```python
from build123d import *

# Parameters (mm, degrees)
SKETCH1_R           = 25.4
SKETCH1_R_2         = 1.5
SKETCH1_R_3         = 12.7
BOSS_EXTRUDE1_DEPTH = 0.396875


with BuildPart() as part:
    # Sketch1 → Boss-Extrude1 (new body)
    with BuildSketch(Plane.XY):
        Circle(SKETCH1_R)
        with Locations((-15.5, 0)):
            Circle(SKETCH1_R_2, mode=Mode.SUBTRACT)
        with Locations((-7.75, 13.423393759)):
            Circle(SKETCH1_R_2, mode=Mode.SUBTRACT)
        with Locations((7.75, 13.423393759)):
            Circle(SKETCH1_R_2, mode=Mode.SUBTRACT)
        with Locations((15.5, 0)):
            Circle(SKETCH1_R_2, mode=Mode.SUBTRACT)
        with Locations((7.75, -13.423393759)):
            Circle(SKETCH1_R_2, mode=Mode.SUBTRACT)
        with Locations((-7.75, -13.423393759)):
            Circle(SKETCH1_R_2, mode=Mode.SUBTRACT)
        Circle(SKETCH1_R_3, mode=Mode.SUBTRACT)
        with BuildLine():
            Line((-1.58439638, 16.926006266), (-1.58439638, 22.168453106))
            ThreePointArc((-1.58439638, 22.168453106), (-11.1125, 19.247414599), (-18.406245362, 12.456354068))
            Line((-18.406245362, 12.456354068), (-13.866153221, 9.835130648))
            ThreePointArc((-13.866153221, 9.835130648), (-13.876900865, 9.842174678), (-13.88768889, 9.849154838))
            ThreePointArc((-13.88768889, 9.849154838), (-8.512839622, 14.744670742), (-1.58577385, 16.951668798))
            ThreePointArc((-1.58577385, 16.951668798), (-1.585122867, 16.938836014), (-1.58439638, 16.926006266))
        make_face(mode=Mode.SUBTRACT)
        with BuildLine():
            Line((1.58439638, 16.926006266), (1.58439638, 22.168453106))
            ThreePointArc((1.58439638, 22.168453106), (11.1125, 19.247414599), (18.406245362, 12.456354068))
            Line((18.406245362, 12.456354068), (13.866153221, 9.835130648))
            ThreePointArc((13.866153221, 9.835130648), (13.876900865, 9.842174678), (13.88768889, 9.849154838))
            ThreePointArc((13.88768889, 9.849154838), (8.512839622, 14.744670742), (1.58577385, 16.951668798))
            ThreePointArc((1.58577385, 16.951668798), (1.585122867, 16.938836014), (1.58439638, 16.926006266))
        make_face(mode=Mode.SUBTRACT)
        with BuildLine():
            Line((15.450549601, 7.090875618), (19.990641742, 9.712099038))
            ThreePointArc((19.990641742, 9.712099038), (22.225, 0), (19.990641742, -9.712099038))
            Line((19.990641742, -9.712099038), (15.450549601, -7.090875618))
            ThreePointArc((15.450549601, -7.090875618), (15.462023732, -7.096661336), (15.47346274, -7.10251396))
            ThreePointArc((15.47346274, -7.10251396), (17.025679244, 0), (15.47346274, 7.10251396))
            ThreePointArc((15.47346274, 7.10251396), (15.462023732, 7.096661336), (15.450549601, 7.090875618))
        make_face(mode=Mode.SUBTRACT)
        with BuildLine():
            Line((-15.450549601, 7.090875618), (-19.990641742, 9.712099038))
            ThreePointArc((-19.990641742, 9.712099038), (-22.225, 0), (-19.990641742, -9.712099038))
            Line((-19.990641742, -9.712099038), (-15.450549601, -7.090875618))
            ThreePointArc((-15.450549601, -7.090875618), (-15.462023732, -7.096661336), (-15.47346274, -7.10251396))
            ThreePointArc((-15.47346274, -7.10251396), (-17.025679244, 0), (-15.47346274, 7.10251396))
            ThreePointArc((-15.47346274, 7.10251396), (-15.462023732, 7.096661336), (-15.450549601, 7.090875618))
        make_face(mode=Mode.SUBTRACT)
        with BuildLine():
            Line((-13.866153221, -9.835130648), (-18.406245362, -12.456354068))
            ThreePointArc((-18.406245362, -12.456354068), (-11.1125, -19.247414599), (-1.58439638, -22.168453106))
            Line((-1.58439638, -22.168453106), (-1.58439638, -16.926006266))
            ThreePointArc((-1.58439638, -16.926006266), (-1.585122867, -16.938836014), (-1.58577385, -16.951668798))
            ThreePointArc((-1.58577385, -16.951668798), (-8.512839622, -14.744670742), (-13.88768889, -9.849154838))
            ThreePointArc((-13.88768889, -9.849154838), (-13.876900865, -9.842174678), (-13.866153221, -9.835130648))
        make_face(mode=Mode.SUBTRACT)
        with BuildLine():
            Line((1.58439638, -16.926006266), (1.58439638, -22.168453106))
            ThreePointArc((1.58439638, -22.168453106), (11.1125, -19.247414599), (18.406245362, -12.456354068))
            Line((18.406245362, -12.456354068), (13.866153221, -9.835130648))
            ThreePointArc((13.866153221, -9.835130648), (13.876900865, -9.842174678), (13.88768889, -9.849154838))
            ThreePointArc((13.88768889, -9.849154838), (8.512839622, -14.744670742), (1.58577385, -16.951668798))
            ThreePointArc((1.58577385, -16.951668798), (1.585122867, -16.938836014), (1.58439638, -16.926006266))
        make_face(mode=Mode.SUBTRACT)
    extrude(amount=BOSS_EXTRUDE1_DEPTH)


solid = part.part
```
CAD build for the part. Positions are in the model's coordinates, mm. Give positions to 0.01 mm unless a question says otherwise; leave off trailing zeros. Loops run counter-clockwise (first coordinate to the right, second up) from the corner with the lowest first, then second, coordinate; pieces in that order, holes last. Notation, with made-up numbers: M 72.5,22.5 L 113.5,22.5 A9 cw 113.5,27.5 Z; hole C -22.5,-15.75 d8. An arc over 180 degrees is marked long. Use one line per item in the form item = value.
Item 1: Slice it at A-A (y = 0). List the corners of the cut face in (x, z) (3 decimals).
Determined:
outline = M -25.4,0 L -22.225,0 L -22.225,0.397 L -25.4,0.397 Z; M -17.026,0 L -17,0 L -17,0.397 L -17.026,0.397 Z; M -14,0 L -12.7,0 L -12.7,0.397 L -14,0.397 Z; M 12.7,0 L 14,0 L 14,0.397 L 12.7,0.397 Z; M 17,0 L 17.026,0 L 17.026,0.397 L 17,0.397 Z; M 22.225,0 L 25.4,0 L 25.4,0.397 L 22.225,0.397 Z
Item 2: Slice it at B-B (x = -7.75). List the corners of the cut face in (y, z), plus the area to 3 significant figures.
Determined:
outline = M -24.19,0 L -20.83,0 L -20.83,0.4 L -24.19,0.4 Z; M -15.16,0 L -14.92,0 L -14.92,0.4 L -15.16,0.4 Z; M -11.92,0 L -10.06,0 L -10.06,0.4 L -11.92,0.4 Z; M 10.06,0 L 11.92,0 L 11.92,0.4 L 10.06,0.4 Z; M 14.92,0 L 15.16,0 L 15.16,0.4 L 14.92,0.4 Z; M 20.83,0 L 24.19,0 L 24.19,0.4 L 20.83,0.4 Z
area = 4.33 mm2
Item 3: Two-plate mould, pull along Y, no slides. Class faces 1 (the face through (10.99, -19.317, 0.196)), 2 (the face through (-12, -5, 0)), 3 (the face through (-5.506, -24.796, 0.196)): pulls with the +Y half, pulls with the -Y half, needs draft (parallel to the pull), parting line crosses it, or undercut.
Determined:
face_1 = undercut
face_2 = needs draft
face_3 = parting line crosses it
Item 4: Slice it at C-C (x = 0). List the corners of the cut face in (y, z), plus the area to 3 significant figures.
Determined:
outline = M -25.4,0 L -12.7,0 L -12.7,0.4 L -25.4,0.4 Z; M 12.7,0 L 25.4,0 L 25.4,0.4 L 12.7,0.4 Z
area = 10.1 mm2
Item 5: Drill centre lines: probe 1 along Y at (x, z) = (7, 0.35); probe 2 along X at (y, z) = (10, 0.1); probe 3 along X at (y, z) = (-14, 0.1). Where is each one in solid material? Low to high. Write a range as from..to.
Determined:
probe_1 = -24.42..-21.09, -15.52..-14.72, -12.12..-10.6, 10.6..12.12, 14.72..15.52, 21.09..24.42
probe_2 = -23.35..-14.15, -13.78..-7.83, 7.83..13.78, 14.15..23.35
probe_3 = -21.19..-17.26, -9.69..-9.13, -6.37..6.37, 9.13..9.69, 17.26..21.19
Item 6: Flat gauge pins, fed straight in: pin 1 (2.5 mm diameter, centred on x = 7.75, y = 13.42, fed in from -Z); pin 2 (5 mm diameter, centred on x = -15.5, y = 0, fed in from -Z). Where does each tip first touch, or does it go through?
Determined:
pin_1 = through
pin_2 = 0
Item 7: Slice it at D-D (y = 9). List the corners of the cut face in (x, z).
Determined:
outline = M -23.75,0 L -20.32,0 L -20.32,0.4 L -23.75,0.4 Z; M -18.76,0 L -8.96,0 L -8.96,0.4 L -18.76,0.4 Z; M 8.96,0 L 18.76,0 L 18.76,0.4 L 8.96,0.4 Z; M 20.32,0 L 23.75,0 L 23.75,0.4 L 20.32,0.4 Z
